```python
from build123d import *

# Parameters (mm, degrees)
SKETCH2_W           = 113.03
SKETCH2_H           = 100.33
BOSS_EXTRUDE1_DEPTH = 2.54
FILLET1_R           = 2.54
FILLET2_R           = 2.54
CUT_EXTRUDE1_DEPTH  = 3.54
SKETCH5_R           = 3.175
CUT_EXTRUDE2_DEPTH  = 3.54
CUT_EXTRUDE3_DEPTH  = 3.54
SKETCH9_R           = 1.905
CUT_EXTRUDE4_DEPTH  = 5.08


with BuildPart() as part:
    # Sketch2 → Boss-Extrude1 (new body)
    with BuildSketch(Plane(origin=(0, 0, 0), x_dir=(1, 0, 0), z_dir=(0, 1, 0))):
        Rectangle(SKETCH2_W, SKETCH2_H)
    extrude(amount=BOSS_EXTRUDE1_DEPTH)

    # Fillet1
    fillet1_edges = [part.edges().sort_by_distance(p)[0] for p in [
        (-56.515, 1.27, -50.165),
    ]]
    fillet(fillet1_edges, radius=FILLET1_R)

    # Fillet2
    fillet2_edges = [part.edges().sort_by_distance(p)[0] for p in [
        (56.515, 1.27, 50.165),
        (-56.515, 1.27, 50.165),
        (56.515, 1.27, -50.165),
    ]]
    fillet(fillet2_edges, radius=FILLET2_R)

    # Sketch4 → Cut-Extrude1 (cut, through all)
    with BuildSketch(Plane(origin=(0, 2.54, 0), x_dir=(1, 0, 0), z_dir=(0, 1, 0))):
        Polygon((-37.461428175, 50.165), (0, 16.968868313), (37.461428175, 50.165), align=None)
        Polygon((0, -16.968868313), (37.461428175, -50.165), (-37.461428175, -50.165), align=None)
        Polygon((-56.515, 36.721051224), (-19.783044536, -0.01090424), (-56.515, -36.742859704), align=None)
        Polygon((19.783044536, -0.01090424), (56.515, -36.742859704), (56.515, 36.721051224), align=None)
    extrude(amount=-CUT_EXTRUDE1_DEPTH, mode=Mode.SUBTRACT)

    # Sketch5 → Cut-Extrude2 (cut, through all)
    with BuildSketch(Plane(origin=(0, 2.54, 0), x_dir=(1, 0, 0), z_dir=(0, 1, 0))):
        with Locations((-50.345804437, 44.613514098)):
            Circle(SKETCH5_R)
        with Locations((49.165550163, -43.56764163)):
            Circle(SKETCH5_R)
        with Locations((51.157011398, 45.33235837)):
            Circle(SKETCH5_R)
        with Locations((-49.976757123, -44.286485902)):
            Circle(SKETCH5_R)
    extrude(amount=-CUT_EXTRUDE2_DEPTH, mode=Mode.SUBTRACT)

    # Sketch8 → Cut-Extrude3 (cut, through all)
    with BuildSketch(Plane(origin=(0, 2.54, 0), x_dir=(1, 0, 0), z_dir=(0, 1, 0))):
        Polygon((-15.34300557, 0.671713564), (17.39574797, -29.394488667), (31.140297562, -14.428201334), (-1.598455979, 15.638000897), align=None)
    extrude(amount=-CUT_EXTRUDE3_DEPTH, mode=Mode.SUBTRACT)

    # Sketch9 → Cut-Extrude4 (cut)
    with BuildSketch(Plane(origin=(0, 2.54, 0), x_dir=(1, 0, 0), z_dir=(0, 1, 0))):
        with Locations((22.938442662, -27.1142567)):
            Circle(SKETCH9_R)
        with Locations((29.632724368, -19.812515234)):
            Circle(SKETCH9_R)
        with Locations((-13.541882712, 6.388082929)):
            Circle(SKETCH9_R)
        with Locations((-6.83523338, 13.678466371)):
            Circle(SKETCH9_R)
    extrude(amount=-CUT_EXTRUDE4_DEPTH, mode=Mode.SUBTRACT)


solid = part.part
```
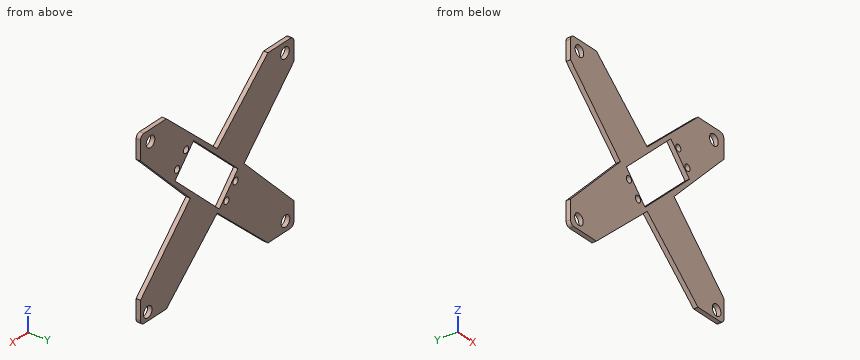
For this review, take the finished solid that the model builds, in its own axes (mm). Round coordinates to 2 decimals unless told otherwise and drop trailing zeros. Write each loop counter-clockwise with the first axis right and the second up, starting at its lowest first coordinate (ties: lowest second). Pieces come first, ordered by that corner, then holes. Notation, with made-up numbers: (40.25, 76.25) -> (65.25, 76.25) arc R18 ccw to (65.25, 104.25) -> close; hole circle Ø11 at (57.25, 48.5). An arc over 180 degrees is marked (long way). Use one line per item in the form item = value.
Q1. Consider section A-A (x = 43.5). State the section outline as (y, z) points (3 decimals), then the cut area to 3 significant figures.
Resolved:
outline = (0, -50.165) -> (2.54, -50.165) -> (2.54, -23.706) -> (0, -23.706) -> close; (0, 23.728) -> (2.54, 23.728) -> (2.54, 50.165) -> (0, 50.165) -> close
area = 134 mm²
Q2. Clearance check with flat-ended pins moving along their axes: pin 1 Ø4 at (x, z) = (49.17, 43.57) entering from +Y; pin 2 Ø1 at (x, y) = (-14.5, 1) entering from -Z; pin 3 Ø1 at (y, z) = (0.5, -35) entering from +X; pin 4 Ø1 at (y, z) = (2, -29) entering from -X. State where each tip first meets the part, or that it passes through.
Resolved:
pin_1 = through
pin_2 = -30.26
pin_3 = 55.29
pin_4 = -49.29
Q3. Consider section C-C (x = -13.5). State the section outline as (y, z) points.
Resolved:
outline = (0, -28.93) -> (2.54, -28.93) -> (2.54, -8.29) -> (0, -8.29) -> close; (0, -4.48) -> (2.54, -4.48) -> (2.54, -2.68) -> (0, -2.68) -> close; (0, 1.02) -> (2.54, 1.02) -> (2.54, 28.93) -> (0, 28.93) -> close
Q4. Consider section D-D (y = 1.5). State how many separate pieces and enclosed holes the cut face has, then the cut area to 3 significant figures.
Resolved:
separate_pieces = 1
enclosed_holes = 9
area = 5,070 mm²
Q5. To check wall thickness, follow probe 1 along X at (y, z) = (1.9, 44) (3 decimals); probe 2 along Z at (x, y) = (-52, 1.5) (3 decimals); probe 3 along Z at (x, y) = (46.5, 0.2) (3 decimals). State the ranges of each line that lie inside material, in increasing order. Write a range as from..to.
Resolved:
probe_1 = -56.515..-53.139, -46.815..-30.504, 30.504..46.02, 52.311..56.515
probe_2 = -50.165..-47.324, -41.903..-32.206, 32.228..41.84, 46.733..50.165
probe_3 = -50.165..-26.706, 26.728..41.843, 45.293..50.165
Q6. Consider section B-B (z = -27). State the section outline as (x, y) points.
Resolved:
outline = (-46.79, 0) -> (-11.32, 0) -> (-11.32, 2.54) -> (-46.79, 2.54) -> close; (11.32, 0) -> (46.79, 0) -> (46.79, 2.54) -> (11.32, 2.54) -> close
